CAD build for the part. Positions are in the model's coordinates, mm. A direction names the side the tool comes from. Round coordinates to 2 decimals unless told otherwise and drop trailing zeros. Write each loop counter-clockwise with the first axis right and the second up, starting at its lowest first coordinate (ties: lowest second). Pieces come first, ordered by that corner, then holes. Notation, with made-up numbers: (37, 50) - (44, 50) arc R22 ccw to (44, 59) - close; hole circle Ø10 at (54.5, 70). An arc over 180 degrees is marked (long way). Answer in a Markdown table with one row per item.
```python
from build123d import *

# Parameters (mm, degrees)
SKETCH1_W           = 50
SKETCH1_H           = 840
BOSS_EXTRUDE1_DEPTH = 3
SKETCH2_W           = 23
SKETCH2_H           = 840
BOSS_EXTRUDE2_DEPTH = 30
SKETCH3_W           = 3
SKETCH3_H           = 840
CUT_EXTRUDE1_DEPTH  = 30


with BuildPart() as part:
    # Sketch1 → Boss-Extrude1 (new body)
    with BuildSketch(Plane.XY):
        with Locations((25, -420)):
            Rectangle(SKETCH1_W, SKETCH1_H)
    extrude(amount=BOSS_EXTRUDE1_DEPTH)

    # Sketch2 → Boss-Extrude2 (add)
    with BuildSketch(Plane.XY.offset(3)):
        with Locations((25, -420)):
            Rectangle(SKETCH2_W, SKETCH2_H)
    extrude(amount=BOSS_EXTRUDE2_DEPTH)

    # Sketch3 → Cut-Extrude1 (cut)
    with BuildSketch(Plane.XY.offset(33)):
        with Locations((25, -420)):
            Rectangle(SKETCH3_W, SKETCH3_H)
    extrude(amount=-CUT_EXTRUDE1_DEPTH, mode=Mode.SUBTRACT)


solid = part.part
```
Q1. Pull direction X, two halves, no side cores. Call faces 4 (the flat face through (25, -414, 0)), 5 (the flat face through (23.5, -426, 18)), 6 (the flat face through (13.5, -426, 18)): released by +X, released by -X, zero draft, split by the parting line, or undercut.
Computed:
| item | result |
|---|---|
| face 4 | zero draft |
| face 5 | undercut |
| face 6 | released by -X |
Q2. Drill centre lines: line 1 (X direction, y = -351, z = 5); line 2 (Z direction, x = 37, y = -137.5). Where is each one in solid material? Low to high.
Computed:
| item | result |
|---|---|
| line 1 | x = 13.5 to 23.5, 26.5 to 36.5 |
| line 2 | z = 0 to 3 |
Q3. 3-axis set-ups, long thin cutter, end or side, ignore diameter. For faces 1 (the flat face through (7, -414, 3)), 2 (the flat face through (43, -414, 3)), 3 (the flat face through (26.5, -426, 18)): which of +Z, -Z, +X, -X, +Y, -Y reach the whole face in a straight line?
Computed:
| item | result |
|---|---|
| face 1 | +Z, -X, +Y, -Y |
| face 2 | +Z, +X, +Y, -Y |
| face 3 | +Z, +Y, -Y |
Q4. Flat gauge pins, fed straight in: pin 1 (11 mm diameter, centred on x = 43, y = -211, fed in from +Z); pin 2 (12 mm diameter, centred on y = -487, z = 14.5, fed in from +X); pin 3 (4 mm diameter, centred on y = -635.5, z = 28.5, fed in from -X). Where does each tip first touch, or does it go through?
Computed:
| item | result |
|---|---|
| pin 1 | stops at z = 3 |
| pin 2 | stops at x = 36.5 |
| pin 3 | stops at x = 13.5 |
Q5. Saw through at B-B on y = -359. List the corners of the cut face in (x, z).
Computed:
| item | result |
|---|---|
| outline | (0, 0) - (50, 0) - (50, 3) - (36.5, 3) - (36.5, 33) - (26.5, 33) - (26.5, 3) - (23.5, 3) - (23.5, 33) - (13.5, 33) - (13.5, 3) - (0, 3) - close |
Q6. Saw through at A-A on z = 12. List the corners of the cut face in (x, y), then the cut area to 3 significant figures.
Computed:
| item | result |
|---|---|
| outline | (13.5, -840) - (23.5, -840) - (23.5, 0) - (13.5, 0) - close; (26.5, -840) - (36.5, -840) - (36.5, 0) - (26.5, 0) - close |
| area | 16,800 mm2 |
